Autodesk Inventor part; units mm, degrees
ref_plane "YZ Plane" through (0, 0, 0) normal (1, 0, 0) x (0, 1, 0)
ref_plane "XZ Plane" through (0, 0, 0) normal (0, 1, 0) x (-1, 0, 0)
ref_plane "XY Plane" through (0, 0, 0) normal (0, 0, 1) x (1, 0, 0)
sketch "Sketch1" plane through (0, 0, 0) normal (0, 1, 0) x (-1, 0, 0)
  arc A0 (-25, 0) -> (0, 0) centre (-12.5, 15.6125) ccw
  arc A1 (0, 0) -> (-25, 0) centre (-12.5, -8.2916) ccw
  dimension "d0" = 25
  dimension "d1" = 20
  dimension "d2" = 15
extrude "Extrusion1" add sketch "Sketch1" along normal blind 1
fillet "Fillet1" radius 2 2 edges at (25, 0.5, 0) (0, 0.5, 0)
sketch "Sketch2" plane through (0, 1, 0) normal (0, 1, 0) x (1, 0, 0)
  arc A0 (1.3645, -1.7583) -> (23.6355, -1.7583) centre (12.5, 8.2916) ccw
  arc A1 (1.3645, -1.7583) -> (23.6355, -1.7583) centre (12.5, 8.2916) ccw
  arc A2 (9.4548, -6.3961) -> (12.5, -5.3578) centre (10.2741, -3.8143) ccw
  arc A3 (12.5, -5.3578) -> (15.5452, -6.3961) centre (14.7259, -3.8143) ccw
  line L0 (9.4548, -6.3961) -> (10.705, -7.1711)
  line L1 (10.705, -7.1711) -> (14.8328, -7.2667)
  line L2 (14.8328, -7.2667) -> (15.5452, -6.3961)
  point P0 (0, 0)
extrude "Extrusion2" cut sketch "Sketch2" against normal blind 1 contours A2 A0 A3 L2 L1 L0 | A2 A3 A0
sketch "Sketch3" plane through (0, 1, 0) normal (0, 1, 0) x (1, 0, 0)
  arc A0 (1.7769, 1.2699) -> (1.3645, -1.7583) centre (2.8492, -0.4183) ccw
  line L0 (0.8935, 0) -> (2.3935, 0)
  arc A1 (23.6355, -1.7583) -> (23.2231, 1.2699) centre (22.1508, -0.4183) ccw
  line L1 (24.1065, 0) -> (22.6065, 0)
  circle A2 centre (2.3935, 0) radius 0.75
  circle A3 centre (22.6065, 0) radius 0.75
  circle A4 centre (11.6968, 3.0289) radius 0.5
  point P0 (0, 0)
  dimension "d10" = 1.5
  dimension "d11" = 1.5
  dimension "d12" = 1.5
  dimension "d13" = 1.5
  dimension "d14" = 1
extrude "Extrusion3" cut sketch "Sketch3" against normal blind 1
sketch "Sketch4" plane through (0, 1, 0) normal (0, 1, 0) x (1, 0, 0)
  circle A0 centre (12.5028, -4.4622) radius 0.5
  point P0 (0, 0)
  dimension "d17" = 1
extrude "Extrusion4" cut sketch "Sketch4" against normal blind 1
properties part number "nariz"
For this review, take the finished solid that the model builds, in its own axes (mm). Round coordinates to 2 decimals unless told otherwise and drop trailing zeros. Loops run counter-clockwise (first coordinate to the right, second up) from the corner with the lowest first, then second, coordinate; pieces in that order, holes last.
Q1. Add section D-D on x = 15.75. Write out the cut boundary in (y, z).
Result sheet:
outline: (0, -4.12) - (1, -4.12) - (1, 6.35) - (0, 6.35) - close
Q2. To check wall thickness, follow line 1 along X through (y, z) = (0.5, 0.5); line 2 along X through (y, z) = (0.8, 0); line 3 along Z through (x, y) = (12.75, 0.8). State the ranges of each line that lie inside material, in increasing order.
Result sheet:
line 1: x = 0.85 to 1.83, 2.95 to 22.05, 23.17 to 24.15
line 2: x = 0.89 to 1.64, 3.14 to 21.86, 23.36 to 24.11
line 3: z = -4.39 to 4.03, 4.9 to 5.67
Q3. Add section A-A on z = 0. Give the number of separate pieces and of enclosed holes in the cut face, plus the area to 3 significant figures.
Result sheet:
separate pieces: 3
enclosed holes: 0
area: 20.2 mm2
Q4. Mouldability with a two-part tool opening along X and no side actions: class faces 1 (the face through (12.342, 0.493, -4.387)), 2 (the face through (12.16, 0.51, -2.84)), 3 (the face through (12.438, 0.507, 3.966)), 4 (the face through (19.73, 0.49, 4.85)) as +X half, -X half, draft (parallel to the pull), parting line (faces both ways), or undercut.
Result sheet:
face 1: parting line
face 2: undercut
face 3: undercut
face 4: +X half
Q5. Insertion check: pin 1 Ø1.2 at (x, z) = (2.39, 0) entering from +Y; pin 2 Ø1 at (x, z) = (11, 5) entering from -Y. Each pin has a flat end and moves straight along its axis. Give the tip position at first contact, or say it passes through.
Result sheet:
pin 1: passes through
pin 2: stops at y = 0
Q6. Add section C-C on z = 3. Write out the cut boundary in (x, y), plus the area to 3 significant figures.
Result sheet:
outline: (2.63, 0) - (22.37, 0) - (22.37, 1) - (2.63, 1) - close
area: 19.7 mm2
